CAD build for the part. Positions are in the model's coordinates, mm. A direction names the side the tool comes from. Give positions to 0.01 mm unless a question says otherwise; leave off trailing zeros. Write each loop counter-clockwise with the first axis right and the second up, starting at its lowest first coordinate (ties: lowest second). Pieces come first, ordered by that corner, then holes. Notation, with made-up numbers: (33, 12) -> (91, 12) arc R20 cw to (91, 46) -> close; hole circle Ø2 at (-2.75, -6). An arc over 180 degrees is marked (long way). Answer in a Markdown table with one row per item. Add a question column.
```python
from build123d import *

# Parameters (mm, degrees)
F0_W     = 20
F0_H     = 25
F0_R     = 3.5
F1_DEPTH = 10


with BuildPart() as f1:
    # F0 (on Top) → F1 (new body)
    with BuildSketch(Plane.XY):
        with Locations((-35.199998, 27.2)):
            Rectangle(F0_W, F0_H)
        with Locations((-39.446462, 33.300817)):
            Circle(F0_R, mode=Mode.SUBTRACT)
        Polygon((-5.199998, -5.3), (-45.199998, -5.3), (-45.199998, -25.3), (14.800002, -25.3), (14.800002, -5.3), align=None)
        with Locations((6.069177, -12.224216)):
            Circle(F0_R, mode=Mode.SUBTRACT)
        Polygon((-25.199998, 14.7), (-45.199998, 14.7), (-45.199998, -5.3), (-5.199998, -5.3), (-5.199998, 14.7), align=None)
    extrude(amount=F1_DEPTH)


solid = f1.part
```
Item 1: Drop flat-ended pins along their axis: pin 1 Ø6.5 at (x, y) = (-39.45, 33.3) entering from +Z (1 decimal); pin 2 Ø3 at (x, z) = (-14.5, 7.5) entering from +Y. Give the stop position or say it passes through.
Item 2: Slice it at A-A, the plane y = -13.5. List the corners of the cut face in (x, z), then the cut area to 3 significant figures.
Item 3: Slice it at B-B, the plane x = 5. List the corners of the cut face in (y, z).
Item 4: Slice it at D-D, the plane y = 8.5. List the corners of the cut face in (x, z), then the cut area to 3 significant figures.
Item 5: Slice it at C-C, the plane z = 5.5. List the corners of the cut face in (x, y).
Item 6: Mould opens along X. For faces 3 (the face through (5.614, -8.754, 4.93)), 4 (the face through (-22, 0, 10)), 5 (the face through (-45.2, 8, 5)) say: released by +X, released by -X, zero draft, split by the parting line, or undercut.
Item 7: Which spindle directions (+Z, -Z, +X, -X, +Y, -Y) get a long thin tool onto all of the face, cutting with end or side? Do faces 1 (the face through (-5.2, 5, 5)), 2 (the face through (-22, 0, 0)). Say none if no direction does.
Item 8: Probe L1, parallel to X at y = 12, z = 2; L2, parallel to Y at x = 12.5, z = 1.5; L3, parallel to X at y = -12, z = 5.5. List the from-to ranges inside material, lowest first. Write a range as from..to.
Answer key:
| question | item | result |
|---|---|---|
| 1 | pin 1 | passes through |
| 1 | pin 2 | stops at y = 14.7 |
| 2 | outline | (-45.2, 0) -> (2.81, 0) -> (2.81, 10) -> (-45.2, 10) -> close; (9.33, 0) -> (14.8, 0) -> (14.8, 10) -> (9.33, 10) -> close |
| 2 | area | 535 mm² |
| 3 | outline | (-25.3, 0) -> (-15.56, 0) -> (-15.56, 10) -> (-25.3, 10) -> close; (-8.89, 0) -> (-5.3, 0) -> (-5.3, 10) -> (-8.89, 10) -> close |
| 4 | outline | (-45.2, 0) -> (-5.2, 0) -> (-5.2, 10) -> (-45.2, 10) -> close |
| 4 | area | 400 mm² |
| 5 | outline | (-45.2, -25.3) -> (14.8, -25.3) -> (14.8, -5.3) -> (-5.2, -5.3) -> (-5.2, 14.7) -> (-25.2, 14.7) -> (-25.2, 39.7) -> (-45.2, 39.7) -> close; hole circle Ø7 at (-39.45, 33.3); hole circle Ø7 at (6.07, -12.22) |
| 6 | face 3 | undercut |
| 6 | face 4 | zero draft |
| 6 | face 5 | released by -X |
| 7 | face 1 | +Z, -Z, +X, +Y |
| 7 | face 2 | -Z, +X, -X, +Y, -Y |
| 8 | L1 | x = -45.2..-5.2 |
| 8 | L2 | y = -25.3..-5.3 |
| 8 | L3 | x = -45.2..2.58, 9.56..14.8 |
